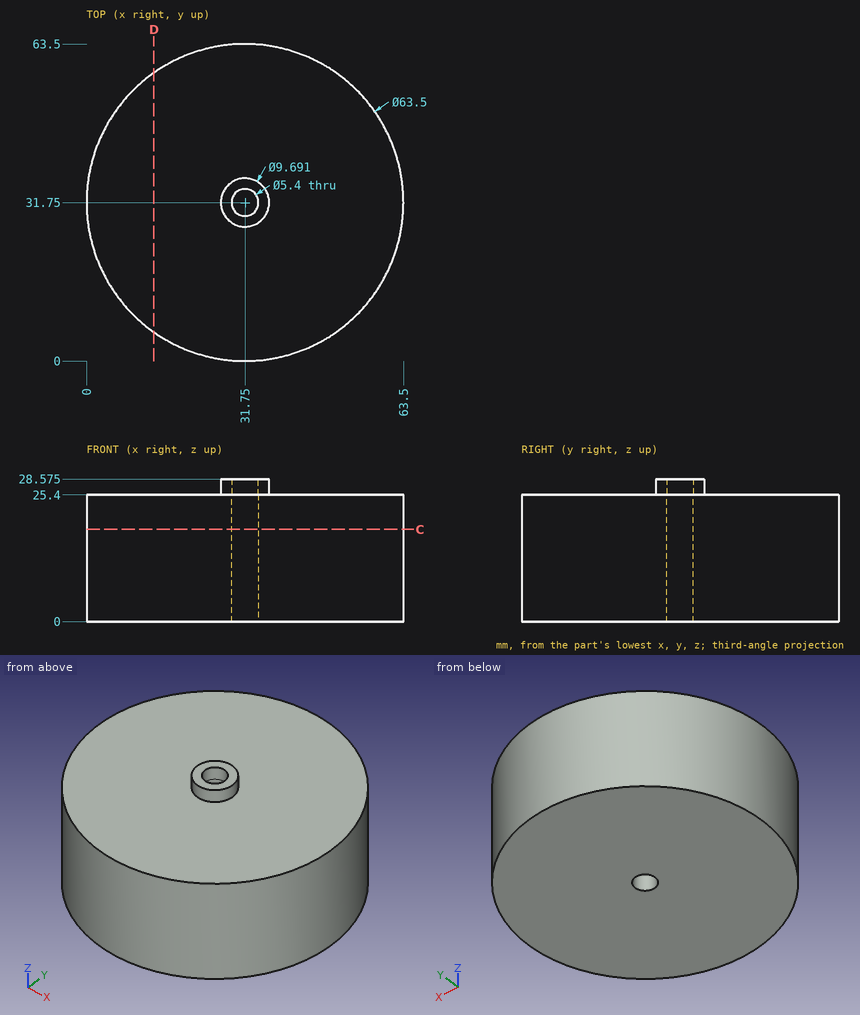
Study the drawing (mm; zero at the part's minimum x, y, z) and answer. Give positions to 0.01 mm unless a question says otherwise; leave off trailing zeros. Write each loop counter-clockwise with the first axis right and the second up, starting at its lowest first coordinate (ties: lowest second). Pieces come first, ordered by that corner, then holes. Notation, with made-up numbers: (-9, 14.25) - (-2, 14.25) arc R24 cw to (-2, 44.25) - close; hole circle Ø2 at (-14.75, 23). An arc over 180 degrees is marked (long way). Write item = value, one per line. Start each with the question number.
Item 1: Each of these flat-tipped pins is pushed along its axis until it touches: P1, Ø10, axis at x = 39.5, y = 16, coming from the +Z side; P2, Ø2, axis at y = 34.5, z = 22, coming from the -X side; P3, Ø6, axis at y = 17, z = 4, coming from the -X side. Where does it stop, or does it pass through?
Item 2: Find the intervals of material crossed by probe 1 along Y at (x, z) = (31.75, 9.75); probe 2 along Y at (x, z) = (31.75, 26.7); probe 3 along Z at (x, y) = (50, 53), in increasing order. Write a range as [from, to].
Item 3: Find section C-C (z = 18.5). Give the vertices of the cut face in (x, y).
Item 4: Find section D-D (x = 13.5). Give the vertices of the cut face in (y, z).
Response:
q1.P1 = 25.4
q1.P2 = 0.05
q1.P3 = 2.25
q2.probe_1 = [0, 29.05], [34.45, 63.5]
q2.probe_2 = [26.9, 29.05], [34.45, 36.6]
q2.probe_3 = [0, 25.4]
q3.outline = circle Ø63.5 at (31.75, 31.75); hole circle Ø5.4 at (31.75, 31.75)
q4.outline = (5.77, 0) - (57.73, 0) - (57.73, 25.4) - (5.77, 25.4) - close
